```python
from build123d import *

# Parameters (mm, degrees)
SKETCH1_W                = 31
SKETCH1_H                = 80
BOSS_EXTRUDE1_DEPTH      = 2
FILLET1_R                = 15.5
BOSS_EXTRUDE2_DEPTH      = 30
BOSS_EXTRUDE2_DEPTH_BACK = 30
FILLET3_R                = 1


with BuildPart() as part:
    # Sketch1 → Boss-Extrude1 (new body)
    with BuildSketch(Plane.XY):
        Rectangle(SKETCH1_W, SKETCH1_H)
    extrude(amount=BOSS_EXTRUDE1_DEPTH)

    # Fillet1
    fillet1_edges = [part.edges().sort_by_distance(p)[0] for p in [
        (-15.5, 40, 1),
        (15.5, -40, 1),
        (-15.5, -40, 1),
        (15.5, 40, 1),
    ]]
    fillet(fillet1_edges, radius=FILLET1_R - 0.0001)  # a hair under: the kernel refuses the full size

    # Sketch2 → Boss-Extrude2 (add, two sides: drawn at the far end of the back side and taken through both)
    with BuildSketch(Plane(origin=(0, 0, 0), x_dir=(1, 0, 0), z_dir=(0, 1, 0)).offset(-BOSS_EXTRUDE2_DEPTH_BACK)):
        Polygon((-10.5, 0), (-7.5, 0), (-7.5, 2.375), (-6.35, 2.375), (-6.35, 4.75), (-7.5, 4.75), (-10.5, 4.75), (-11.65, 4.75), (-11.65, 2.375), (-10.5, 2.375), align=None)
        Polygon((10.5, 0), (10.5, 2.375), (11.65, 2.375), (11.65, 4.75), (6.35, 4.75), (6.35, 2.375), (7.5, 2.375), (7.5, 0), align=None)
    extrude(amount=BOSS_EXTRUDE2_DEPTH + BOSS_EXTRUDE2_DEPTH_BACK)

    # Fillet3
    fillet3_edges = [part.edges().sort_by_distance(p)[0] for p in [
        (-15.5, 0, 0),
        (-10.960184398, -35.460184398, 0),
        (10.960184398, -35.460184398, 0),
        (15.5, 0, 0),
        (10.960184398, 35.460184398, 0),
        (10.960184398, 35.460184398, 2),
        (15.5, 0, 2),
        (10.960184398, -35.460184398, 2),
        (-10.960184398, -35.460184398, 2),
        (-15.5, 0, 2),
        (-10.960184398, 35.460184398, 0),
        (-10.960184398, 35.460184398, 2),
    ]]
    fillet(fillet3_edges, radius=FILLET3_R - 0.0001)  # a hair under: the kernel refuses the full size


solid = part.part
```
The model under review builds one solid part; all positions refer to its coordinate system, in mm. A direction names the side the tool comes from. Coordinates: 2 decimals unless noted, no trailing zeros. Order: outer loops, then holes, each group sorted by start corner. A loop starts at its lowest first (then second) coordinate and runs counter-clockwise, first axis right, second up. Notation, with made-up numbers: M 15,23.5 L 42,23.5 A30 ccw 42,47.5 Z; hole C -29.75,0.5 d8. An arc over 180 degrees is marked long. One line per question, with ' | ' between items.
(1) For probe 1 along X at (y, z) = (20, -3.25); probe 2 along X at (y, z) = (7, -2); probe 3 along Y at (x, z) = (-10.5, -4), list the stretches that pass through material, from the lowest coordinate up. Write a range as from..to.
Geometry results:
probe 1: x = -11.65..-6.35, 6.35..11.65 | probe 2: x = -10.5..-7.5, 7.5..10.5 | probe 3: y = -30..30
(2) The part is to be moulded in two halves that separate along Z. For faces 6 (the face through (-10.5, 0, -1)), 7 (the face through (-9, -30, -3)), 8 (the face through (-9, 0, -4.75)), say which applies: +Z half, -Z half, draft (parallel to the pull), parting line (faces both ways), or undercut.
Geometry results:
face 6: undercut | face 7: draft | face 8: -Z half
(3) Insertion check: pin 1 (1.4 mm diameter, centred on x = 9.5, z = -2.5, fed in from +Y); pin 2 (2.5 mm diameter, centred on y = -7.5, z = -3.5, fed in from -X); pin 3 (1.4 mm diameter, centred on x = 9.5, z = -2.5, fed in from -Y). Each pin has a flat end and moves straight along its axis. Give the tip position at first contact, or say it passes through.
Geometry results:
pin 1: stops at y = 30 | pin 2: stops at x = -11.65 | pin 3: stops at y = -30
(4) Machinability: for faces 1 (the face through (-11.65, 0, -4)), 2 (the face through (7.5, 0, -1)), 3 (the face through (9, -30, -3)), 4 (the face through (10.5, 0, -1)), 5 (the face through (11.65, 0, -4)), which of the approach directions +Z, -Z, +X, -X, +Y, -Y give a long, thin tool a straight path to every point of the face, cutting with its end or side? Answer none if there is none.
Geometry results:
face 1: -Z, -X, +Y, -Y | face 2: +Y, -Y | face 3: -Z, +X, -X, -Y | face 4: +X, +Y, -Y | face 5: -Z, +X, +Y, -Y
(5) Add section A-A, the plane z = -3.5. Write out the cut boundary in (x, y), then the cut area to 3 significant figures.
Geometry results:
outline: M -11.65,-30 L -6.35,-30 L -6.35,30 L -11.65,30 Z; M 6.35,-30 L 11.65,-30 L 11.65,30 L 6.35,30 Z | area: 636 mm²
